Model file for the job. Use its own axes, mm. A direction names the side the tool comes from. Give positions to 0.01 mm unless a question says otherwise; leave off trailing zeros. Loops run counter-clockwise (first coordinate to the right, second up) from the corner with the lowest first, then second, coordinate; pieces in that order, holes last. Notation, with made-up numbers: M -0.75,-17 L 26.25,-17 A30 cw 26.25,19 Z; hole C 79,21 d11. An arc over 180 degrees is marked long. Answer in a Markdown table with one row per item.
```python
from build123d import *
from build123d import SkipClean  # not in build123d's __all__

# Parameters (mm, degrees)
F0_R      = 25
F1_DEPTH  = 40
F2_R      = 25
F3_DEPTH  = 10
F4_R      = 25
F5_DEPTH  = 10
F7_DEPTH  = 25
F9_DEPTH  = 25
F11_D     = 10
F11_DEPTH = 16.5
F11_TIP   = 3.0043030951


with BuildPart() as f1:
    # F0 (on Front) → F1 (new body, symmetric)
    with BuildSketch(Plane.XZ):
        Polygon((0, 15), (0, 0), (30, 0), (30, 5), (90, 5), (90, 0), (120, 0), (120, 15), (35, 15), align=None)
        with BuildLine():
            Line((56.536927729, 85.2578162484), (35, 15))
            Line((35, 15), (120, 15))
            Line((120, 15), (124.8728873319, 72.0197769993))
            ThreePointArc((124.8728873319, 72.0197769993), (83.3435508402, 40.638805542), (56.536927729, 85.2578162484))
        make_face()
        with BuildLine():
            ThreePointArc((125, 75), (95.186158044, 109.613635532), (56.536927729, 85.2578162484))
            ThreePointArc((56.536927729, 85.2578162484), (83.3435508402, 40.638805542), (124.8728873319, 72.0197769993))
            ThreePointArc((124.8728873319, 72.0197769993), (124.9682073934, 73.5085337111), (125, 75))
        make_face()
        with Locations((90, 75)):
            Circle(F0_R, mode=Mode.SUBTRACT)
    extrude(amount=F1_DEPTH, both=True)

    # F2 (on face) → F3 (cut)
    with BuildSketch(Plane.XZ.offset(40)):
        with BuildLine():
            Line((56.536927729, 85.2578162484), (35, 15))
            Line((35, 15), (120, 15))
            Line((120, 15), (124.8728873319, 72.0197769993))
            ThreePointArc((124.8728873319, 72.0197769993), (96.6564491598, 109.361194458), (56.536927729, 85.2578162484))
        make_face()
        with Locations((90, 75)):
            Circle(F2_R, mode=Mode.SUBTRACT)
    extrude(amount=-F3_DEPTH, mode=Mode.SUBTRACT)

    # F4 (on face) → F5 (cut)
    with BuildSketch(Plane(origin=(0, 40, 0), x_dir=(-1, 0, 0), z_dir=(0, 1, 0))):
        with BuildLine():
            Line((-120, 15), (-35, 15))
            Line((-35, 15), (-56.536927729, 85.2578162484))
            ThreePointArc((-56.536927729, 85.2578162484), (-96.6564491598, 109.361194458), (-124.8728873319, 72.0197769993))
            Line((-124.8728873319, 72.0197769993), (-120, 15))
        make_face()
        with Locations((-90, 75)):
            Circle(F4_R, mode=Mode.SUBTRACT)
    extrude(amount=-F5_DEPTH, mode=Mode.SUBTRACT)

    # F6 (on face) → F7 (cut)
    with BuildSketch(Plane.XZ.offset(30)):
        with BuildLine():
            ThreePointArc((85, 40.3589838486), (60.439413574, 56.2604234265), (56.536927729, 85.2578162484))
            Line((56.536927729, 85.2578162484), (35, 15))
            Line((35, 15), (85, 15))
            Line((85, 15), (85, 40.3589838486))
        make_face()
        with BuildLine():
            Line((120, 15), (124.8728873319, 72.0197769993))
            ThreePointArc((124.8728873319, 72.0197769993), (115.4570862783, 50.980492132), (95, 40.3589838486))
            Line((95, 40.3589838486), (95, 15))
            Line((95, 15), (120, 15))
        make_face()
    with SkipClean():  # cleaning this boolean's faces spoils the solid; the shape is the same uncleaned
        extrude(amount=-F7_DEPTH, mode=Mode.SUBTRACT)

    # F8 (on face) → F9 (cut)
    with BuildSketch(Plane(origin=(0, 30, 0), x_dir=(-1, 0, 0), z_dir=(0, 1, 0))):
        with BuildLine():
            ThreePointArc((-95, 40.3589838486), (-115.4570862783, 50.980492132), (-124.8728873319, 72.0197769993))
            Line((-124.8728873319, 72.0197769993), (-120, 15))
            Line((-120, 15), (-95, 15))
            Line((-95, 15), (-95, 40.3589838486))
        make_face()
        with BuildLine():
            Line((-35, 15), (-56.536927729, 85.2578162484))
            ThreePointArc((-56.536927729, 85.2578162484), (-60.439413574, 56.2604234265), (-85, 40.3589838486))
            Line((-85, 40.3589838486), (-85, 15))
            Line((-85, 15), (-35, 15))
        make_face()
    extrude(amount=-F9_DEPTH, mode=Mode.SUBTRACT)

    # F11
    with Locations(Plane.XY.offset(15)):
        with Locations((15, 25), (15, -25), (105, -25), (105, 25)):
            Hole(F11_D / 2, depth=F11_DEPTH)
            with Locations((0, 0, -(F11_DEPTH + F11_TIP / 2))):  # 118° drill point
                Cone(0, F11_D / 2, F11_TIP, mode=Mode.SUBTRACT)


solid = f1.part
```
(1) Flat gauge pins, fed straight in: P1, Ø2, axis at y = 14, z = 18, coming from the -X side; P2, Ø9, axis at x = 103, z = 33, coming from the -Y side; P3, Ø12, axis at y = 4, z = 47.5, coming from the +X side; P4, Ø8, axis at x = 15, y = -25, coming from the -Z side. Where does each tip first touch, or does it go through?
Established:
| item | result |
|---|---|
| P1 | stops at x = 85 |
| P2 | stops at y = -5 |
| P3 | stops at x = 123.29 |
| P4 | passes through |
(2) Saw through at B-B, the plane y = -25. Give the cut face in (x, z), and give its area (3 significant figures).
Established:
| item | result |
|---|---|
| outline | M 0,0 L 10,0 L 10,15 L 0,15 Z; M 20,0 L 30,0 L 30,5 L 90,5 L 90,0 L 100,0 L 100,15 L 95,15 L 95,40.36 A35 ccw long 85,40.36 L 85,15 L 20,15 Z; M 110,0 L 120,0 L 120,15 L 110,15 Z; hole C 90,75 d50 |
| area | 3,340 mm2 |
(3) Which spindle directions (+Z, -Z, +X, -X, +Y, -Y) get a long thin tool onto all of the face, cutting with end or side? Do faces 1 (the flat face through (85, 18, 28)), 2 (the cylindrical face through (100.381, -26.915, 7.395)), 3 (the flat face through (110, -5, 31)), 4 (the flat face through (95, 18, 28)), 5 (the flat face through (90, 30, 49)). Say none if no direction does.
Established:
| item | result |
|---|---|
| face 1 | -X, +Y |
| face 2 | -Z |
| face 3 | +X, -Y |
| face 4 | +X, +Y |
| face 5 | +Z, +X, -X, +Y |
(4) Saw through at A-A, the plane x = 15. Give the cut face in (y, z), and give its area (3 significant figures).
Established:
| item | result |
|---|---|
| outline | M -40,0 L -30,0 L -30,15 L -40,15 Z; M -20,0 L 20,0 L 20,15 L -20,15 Z; M 30,0 L 40,0 L 40,15 L 30,15 Z |
| area | 900 mm2 |
(5) Mould opens along Y. For faces 6 (the cylindrical face through (16.08, -29.88, 7.4)), 7 (the flat face through (30, -1, 2)), 8 (the flat face through (60, 5, 35)) say: pulls with the +Y half, pulls with the -Y half, needs draft (parallel to the pull), parting line crosses it, or undercut.
Established:
| item | result |
|---|---|
| face 6 | undercut |
| face 7 | needs draft |
| face 8 | pulls with the +Y half |
(6) Wall check: L1, parallel to Y at x = 105, z = 10; L2, parallel to X at y = -15, z = 75.5 (3 decimals); L3, parallel to Z at x = 24.5, y = -12.5. Give the ranges that are in metal, low to high.
Established:
| item | result |
|---|---|
| L1 | y = -40 to -30, -20 to 20, 30 to 40 |
| L2 | x = 55.004 to 65.005, 114.995 to 124.996 |
| L3 | z = 0 to 15 |
(7) Saw through at C-C, the plane z = 65.5. Give the cut face in (x, y).
Established:
| item | result |
|---|---|
| outline | M 50.48,-5 L 56.31,-5 L 56.31,-30 L 66.88,-30 L 66.88,30 L 56.31,30 L 56.31,5 L 50.48,5 Z; M 113.12,-30 L 123.69,-30 L 123.69,-5 L 124.32,-5 L 124.32,5 L 123.69,5 L 123.69,30 L 113.12,30 Z |
(8) Saw through at D-D, the plane y = -35. Give the cut face in (x, z).
Established:
| item | result |
|---|---|
| outline | M 0,0 L 30,0 L 30,5 L 90,5 L 90,0 L 120,0 L 120,15 L 0,15 Z |
